Design review of the part built by this model. Coordinates are the model's own, in mm. A direction names the side the tool comes from. Coordinates: 2 decimals unless noted, no trailing zeros. Loops run counter-clockwise (first coordinate to the right, second up) from the corner with the lowest first, then second, coordinate; pieces in that order, holes last. Notation, with made-up numbers: (87.25, -5.75) -> (132.25, -5.75) arc R13 cw to (132.25, 6.25) -> close; hole circle Ø3 at (56, 39.25). An arc over 180 degrees is marked (long way). One line per item, written item: value. Start each with the question number.
1. Add section A-A on x = 23. Write out the cut boundary in (y, z), plus the area to 3 significant figures.
2. Machinability: for faces 1 (the flat face through (29, 2, 0)), 2 (the flat face through (34, 3, 1)), which of the approach directions +Z, -Z, +X, -X, +Y, -Y give a long, thin tool a straight path to every point of the face, cutting with its end or side? Answer none if there is none.
3. For probe 1 along Y at (x, z) = (43.5, 0.4); probe 2 along X at (y, z) = (0.75, 1.7); probe 3 along X at (y, z) = (1.1, 1.7), list the stretches that pass through material, from the lowest coordinate up.
```python
from build123d import *

# Parameters (mm, degrees)
F1_DEPTH = 2
F2_R     = 0.2


with BuildPart() as f1:
    # F0 (on Top) → F1 (new body)
    with BuildSketch(Plane.XY):
        with BuildLine():
            ThreePointArc((2.0172090196, 1.8148367186), (1.3567207288, 0.5204837279), (0, 0))
            Line((0, 0), (60, 0))
            Line((60, 0), (60, 3))
            Line((60, 3), (7.1340496652, 3))
            Line((7.1340496652, 3), (2.0172090196, 1.8148367186))
        make_face()
        with BuildLine():
            ThreePointArc((-0.286715437, 4.0366195626), (-2.023394625, 1.8847733915), (0, 0))
            Line((0, 0), (0, 1.744815443))
            ThreePointArc((0, 1.744815443), (-0.710712171, 2.8197388016), (-0.286715437, 4.0366195626))
        make_face()
        with BuildLine():
            Line((0, 1.744815443), (0, 0))
            ThreePointArc((0, 0), (1.3567207288, 0.5204837279), (2.0172090196, 1.8148367186))
            Line((2.0172090196, 1.8148367186), (1.1959759108, 1.6246226015))
            ThreePointArc((1.1959759108, 1.6246226015), (1.0578352718, 1.5853362888), (0.9164894863, 1.5598879203))
            ThreePointArc((0.9164894863, 1.5598879203), (0.4429542769, 1.5765730666), (0, 1.744815443))
        make_face()
    extrude(amount=F1_DEPTH)

    # F2
    f2_edges = [f1.edges().sort_by_distance(p)[0] for p in [
        (-0.286715, 4.03662, 1),
    ]]
    fillet(f2_edges, radius=F2_R)


solid = f1.part
```
Worked answers:
1. outline: (0, 0) -> (3, 0) -> (3, 2) -> (0, 2) -> close
1. area: 6.00 mm²
2. face 1: -Z, +X, -X, +Y, -Y
2. face 2: +Z, -Z, +X, +Y
3. probe 1: y = 0 to 3
3. probe 2: x = -1.57 to 60
3. probe 3: x = -1.8 to 60
